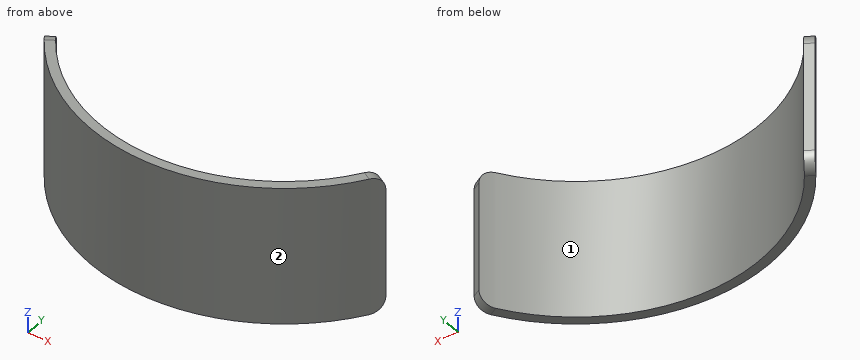
from build123d import *

# Parameters (mm, degrees)
BOSS_EXTRUDE1_DEPTH = 95
FILLET1_R           = 20


with BuildPart() as part:
    # Sketch1 → Boss-Extrude1 (new, symmetric)
    with BuildSketch(Plane.XY):
        with BuildLine():
            Line((-219.970452561, -127), (-230.968975189, -133.35))
            ThreePointArc((-230.968975189, -133.35), (0.181793833, -266.699938041), (231.150554347, -133.035))
            Line((231.150554347, -133.035), (220.143385093, -126.7))
            ThreePointArc((220.143385093, -126.7), (0.173136984, -253.999940991), (-219.970452561, -127))
        make_face()
    extrude(amount=BOSS_EXTRUDE1_DEPTH, both=True)

    # Fillet1
    fillet1_edges = [part.edges().sort_by_distance(p)[0] for p in [
        (225.64696972, -129.8675, 95),
        (225.64696972, -129.8675, -95),
        (-225.469713875, -130.175, -95),
        (-225.469713875, -130.175, 95),
    ]]
    fillet(fillet1_edges, radius=FILLET1_R)


solid = part.part
Read the model definition and answer for the solid it produces. Units are mm, in the model's axes. Face numbers are marked on the shaded views. Coordinates: 2 decimals unless noted, no trailing zeros. Loops run counter-clockwise (first coordinate to the right, second up) from the corner with the lowest first, then second, coordinate; pieces in that order, holes last. Notation, with made-up numbers: (15.25, 10.5) -> (50.25, 10.5) arc R26 ccw to (50.25, 46.5) -> close; hole circle Ø7 at (74, 34). An arc over 180 degrees is marked (long way). Answer in a Markdown table with one row per item.
Item 1: A cutting plane is placed at D-D on x = 59. Determine the outline of the cut face in (y, z), plus the area to 3 significant figures.
Returned:
| item | result |
|---|---|
| outline | (-260.09, -95) -> (-247.05, -95) -> (-247.05, 95) -> (-260.09, 95) -> close |
| area | 2,480 mm^2 |
Item 2: Each of these flat-tipped pins is pushed along its axis until it touches: P1, Ø6, axis at x = 75, y = -239, coming from the -Z side; P2, Ø10, axis at y = -159.5, z = 62.5, coming from the -X side; P3, Ø1.5, axis at y = -141.5, z = -9.5, coming from the -X side; P4, Ø1.5, axis at y = -217.5, z = 65.5, coming from the +X side. Where does it stop, or does it pass through?
Returned:
| item | result |
|---|---|
| P1 | passes through |
| P2 | stops at x = -217.39 |
| P3 | stops at x = -226.54 |
| P4 | stops at x = 155.4 |
Item 3: A cutting plane is placed at A-A on y = -248. Determine the outline of the cut face in (x, z).
Returned:
| item | result |
|---|---|
| outline | (-98.11, -95) -> (-54.88, -95) -> (-54.88, 95) -> (-98.11, 95) -> close; (54.88, -95) -> (98.11, -95) -> (98.11, 95) -> (54.88, 95) -> close |
Item 4: A cutting plane is placed at C-C on y = -201. Determine the outline of the cut face in (x, z).
Returned:
| item | result |
|---|---|
| outline | (-175.29, -95) -> (-155.29, -95) -> (-155.29, 95) -> (-175.29, 95) -> close; (155.29, -95) -> (175.29, -95) -> (175.29, 95) -> (155.29, 95) -> close |
Item 5: For a pull along X with two mould halves and no side action, classify the marked faces 1 and 2 as released by +X, released by -X, zero draft, split by the parting line, or undercut.
Returned:
| item | result |
|---|---|
| face 1 | undercut |
| face 2 | split by the parting line |
Item 6: Straight lines are drawn through the part: line 1 along X through (y, z) = (-177.5, 12); line 2 along X through (y, z) = (-133, 77.5); line 3 along Y through (x, z) = (6, -34). For each, find the intervals that lie inside material, in ascending order. Write a range as [from, to].
Returned:
| item | result |
|---|---|
| line 1 | x = [-199.05, -181.69], [181.69, 199.05] |
| line 2 | x = [-230.05, -216.4], [216.4, 230.78] |
| line 3 | y = [-266.63, -253.93] |
Item 7: A cutting plane is placed at B-B on z = 46. Determine the outline of the cut face in (x, y) (3 decimals).
Returned:
| item | result |
|---|---|
| outline | (-230.969, -133.35) arc R266.7 ccw to (231.151, -133.035) -> (220.143, -126.7) arc R254 cw to (-219.97, -127) -> close |
